```python
from build123d import *
from OCP.BRepFilletAPI import BRepFilletAPI_MakeChamfer

# Parameters (mm, degrees)
SKETCH1_W           = 6.35
SKETCH1_H           = 6.35
SKETCH1_R           = 2.286
BOSS_EXTRUDE1_DEPTH = 6.35
CHAMFER1_SIZE       = 0.79375
CHAMFER1_SIZE2      = 1.374815329
FILLET1_R           = 0.396875
FILLET2_R           = 0.396875


with BuildPart() as part:
    # Sketch1 → Boss-Extrude1 (new body)
    with BuildSketch(Plane(origin=(0, 0, 0), x_dir=(1, 0, 0), z_dir=(0, 1, 0))):
        Rectangle(SKETCH1_W, SKETCH1_H)
        with Locations(Location((0, 0, 0), (0, 0, 270))):
            Circle(SKETCH1_R, mode=Mode.SUBTRACT)
    extrude(amount=BOSS_EXTRUDE1_DEPTH)

    # Chamfer1: one chamfer whose edges measure the first distance from different faces: ONE call of the kernel's chamfer builder (chamfer() names one face for all edges)
    chamfer1_edges_1 = [part.edges().sort_by_distance(p)[0] for p in [
        (3.175, 3.175, 3.175),
    ]]
    chamfer1_side_1 = [part.faces().sort_by_distance(p)[0] for p in [
        (0, 3.175, 3.175),
    ]]
    chamfer1_edges_2 = [part.edges().sort_by_distance(p)[0] for p in [
        (-3.175, 3.175, 3.175),
    ]]
    chamfer1_side_2 = [part.faces().sort_by_distance(p)[0] for p in [
        (-3.175, 3.175, 0),
    ]]
    chamfer1_edges_3 = [part.edges().sort_by_distance(p)[0] for p in [
        (-3.175, 3.175, -3.175),
    ]]
    chamfer1_side_3 = [part.faces().sort_by_distance(p)[0] for p in [
        (0, 3.175, -3.175),
    ]]
    chamfer1_edges_4 = [part.edges().sort_by_distance(p)[0] for p in [
        (3.175, 3.175, -3.175),
    ]]
    chamfer1_side_4 = [part.faces().sort_by_distance(p)[0] for p in [
        (3.175, 3.175, 0),
    ]]
    chamfer1 = BRepFilletAPI_MakeChamfer(part.part.solid().wrapped)
    for e in chamfer1_edges_1:
        chamfer1.Add(CHAMFER1_SIZE, CHAMFER1_SIZE2, e.wrapped, chamfer1_side_1[0].wrapped)  # the first distance lies on this face
    for e in chamfer1_edges_2:
        chamfer1.Add(CHAMFER1_SIZE, CHAMFER1_SIZE2, e.wrapped, chamfer1_side_2[0].wrapped)  # the first distance lies on this face
    for e in chamfer1_edges_3:
        chamfer1.Add(CHAMFER1_SIZE, CHAMFER1_SIZE2, e.wrapped, chamfer1_side_3[0].wrapped)  # the first distance lies on this face
    for e in chamfer1_edges_4:
        chamfer1.Add(CHAMFER1_SIZE, CHAMFER1_SIZE2, e.wrapped, chamfer1_side_4[0].wrapped)  # the first distance lies on this face
    add(Compound.cast(chamfer1.Shape()), mode=Mode.REPLACE)

    # Fillet1
    fillet1_edges = [part.edges().sort_by_distance(p)[0] for p in [
        (-3.175, 6.35, 0.290532664),
        (-0.290532664, 6.35, -3.175),
        (3.175, 6.35, -0.290532664),
        (0.290532664, 6.35, 3.175),
        (-2.487592336, 6.35, 2.778125),
        (2.778125, 6.35, 2.487592336),
        (2.487592336, 6.35, -2.778125),
        (-2.778125, 6.35, -2.487592336),
    ]]
    fillet(fillet1_edges, radius=FILLET1_R)

    # Fillet2
    fillet2_edges = [part.edges().sort_by_distance(p)[0] for p in [
        (0, 0, -2.286),
    ]]
    fillet(fillet2_edges, radius=FILLET2_R)


solid = part.part
```
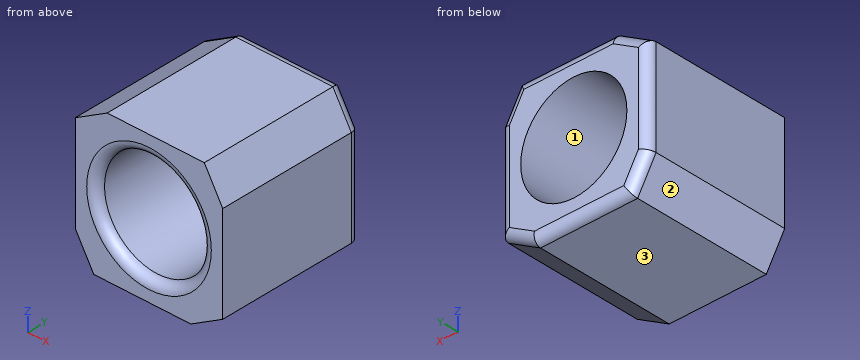
CAD build for the part. Positions are in the model's coordinates, mm. Face numbers are marked on the shaded views. Coordinates: 2 decimals unless noted, no trailing zeros. Order: outer loops, then holes, each group sorted by start corner. A loop starts at its lowest first (then second) coordinate and runs counter-clockwise, first axis right, second up.
(1) Saw through at B-B, the plane x = 0. Write the cut outline in (y, z) (3 decimals).
Solution:
outline: (0, -3.175) - (5.953, -3.175) arc R0.397 ccw to (6.35, -2.778) - (6.35, -2.286) - (0.397, -2.286) arc R0.397 ccw to (0, -2.683) - close; (0, 2.683) arc R0.397 ccw to (0.397, 2.286) - (6.35, 2.286) - (6.35, 2.778) arc R0.397 ccw to (5.953, 3.175) - (0, 3.175) - close
(2) Mould opens along X. For the marked faces 1, 2 and 3 say: released by +X, released by -X, zero draft, split by the parting line, or undercut.
Solution:
face 1: undercut
face 2: released by -X
face 3: zero draft
(3) Drill centre lines: L1, parallel to X at y = 3.7, z = 0 (3 decimals); L2, parallel to X at y = 1.5, z = 1.75 (3 decimals); L3, parallel to Z at x = 0.75, y = 2 (3 decimals). Where is each one in solid material? Low to high.
Solution:
L1: x = -3.175 to -2.286, 2.286 to 3.175
L2: x = -3.175 to -1.471, 1.471 to 3.175
L3: z = -3.175 to -2.159, 2.159 to 3.175
(4) Saw through at A-A, the plane z = 0. Write the cut outline in (x, y) (3 decimals), and give its area (3 significant figures).
Solution:
outline: (-3.175, 0) - (-2.683, 0) arc R0.397 ccw to (-2.286, 0.397) - (-2.286, 6.35) - (-2.778, 6.35) arc R0.397 ccw to (-3.175, 5.953) - close; (2.286, 0.397) arc R0.397 ccw to (2.683, 0) - (3.175, 0) - (3.175, 5.953) arc R0.397 ccw to (2.778, 6.35) - (2.286, 6.35) - close
area: 11.2 mm2
(5) Saw through at C-C, the plane y = 5. Write the cut outline in (x, z) (3 decimals).
Solution:
outline: (-3.175, -1.8) - (-2.381, -3.175) - (1.8, -3.175) - (3.175, -2.381) - (3.175, 1.8) - (2.381, 3.175) - (-1.8, 3.175) - (-3.175, 2.381) - close; hole circle Ø4.572 at (0, 0)
